from build123d import *

# Parameters (mm, degrees)
F0_R     = 8
F1_DEPTH = 350
F4_D     = 5
F4_DEPTH = 16
F4_TIP   = 1.5021515476
F6_D     = 5
F6_DEPTH = 16
F6_TIP   = 1.5021515476


with BuildPart() as f1:
    # F0 (on Front) → F1 (new body)
    with BuildSketch(Plane.XZ):
        Circle(F0_R)
    extrude(amount=F1_DEPTH)

    # F4
    with Locations(Plane(origin=(0, 0, 0), x_dir=(-1, 0, 0), z_dir=(0, 1, 0))):
        with Locations((0, 0)):
            Hole(F4_D / 2, depth=F4_DEPTH)
            with Locations((0, 0, -(F4_DEPTH + F4_TIP / 2))):  # 118° drill point
                Cone(0, F4_D / 2, F4_TIP, mode=Mode.SUBTRACT)

    # F6
    with Locations(Plane.XZ.offset(350)):
        with Locations((0, 0)):
            Hole(F6_D / 2, depth=F6_DEPTH)
            with Locations((0, 0, -(F6_DEPTH + F6_TIP / 2))):  # 118° drill point
                Cone(0, F6_D / 2, F6_TIP, mode=Mode.SUBTRACT)


solid = f1.part
Model file for the job. Use its own axes, mm. Give positions to 0.01 mm unless a question says otherwise; leave off trailing zeros. Order: outer loops, then holes, each group sorted by start corner. A loop starts at its lowest first (then second) coordinate and runs counter-clockwise, first axis right, second up. Notation, with made-up numbers: (-24.5, 76) - (5.5, 76) arc R13 ccw to (5.5, 85) - close; hole circle Ø2 at (79, 9.25). An arc over 180 degrees is marked (long way). Write item = value, one per line. Start each with the question number.
1. Cut at A-A, the plane y = -153. List the corners of the cut face in (x, z), and give its area (3 significant figures).
2. Probe line 1 along Z through (x, y) = (0, -10); line 2 along Z through (x, y) = (-0.75, -185); line 3 along X through (y, z) = (-147.5, 0.25). List the from-to ranges inside material, lowest first.
3. Drop flat-ended pins along their axis: P1, Ø3, axis at x = 0, z = 0, coming from the +Y side; P2, Ø1, axis at x = 1, y = -153.5, coming from the -Z side; P3, Ø4, axis at y = -190, z = 6, coming from the -X side. Give the stop position or say it passes through.
Taken from the geometry:
q1.outline = circle Ø16 at (0, 0)
q1.area = 201 mm²
q2.line_1 = -8 to -2.5, 2.5 to 8
q2.line_2 = -7.96 to 7.96
q2.line_3 = -8 to 8
q3.P1 = -16.6
q3.P2 = -7.98
q3.P3 = -6.93
